from build123d import *

# Parameters (mm, degrees)
BOSS_EXTRUDE1_DEPTH = 45
BOSS_EXTRUDE2_DEPTH = 45


with BuildPart() as part:
    # Sketch1 → Boss-Extrude1 (new body)
    with BuildSketch(Plane(origin=(0, 0, 0), x_dir=(1, 0, 0), z_dir=(0, 1, 0))):
        Polygon((10.257365227, -10.154791575), (13.922990088, 3.805743075), (3.66562486, 13.96053465), (-10.257365227, 10.154791575), (-13.922990088, -3.805743075), (-3.66562486, -13.96053465), align=None)
        Polygon((-2.785874894, -10.610006334), (7.795597573, -7.717641597), (10.581472467, 2.892364737), (2.785874894, 10.610006334), (-7.795597573, 7.717641597), (-10.581472467, -2.892364737), align=None, mode=Mode.SUBTRACT)
    extrude(amount=BOSS_EXTRUDE1_DEPTH)

    # Sketch2 → Boss-Extrude2 (add)
    with BuildSketch(Plane(origin=(0, 45, 0), x_dir=(1, 0, 0), z_dir=(0, 1, 0))):
        Polygon((-6.68367368, -6.751185536), (1.391190433, 10.228779981), (2.592952284, 10.557272411), (-5.972802955, -7.454947554), align=None)
        Polygon((2.504861339, -9.163823965), (3.684441387, 9.720425506), (2.928005116, 10.469297414), (1.68769549, -9.387190014), align=None)
    extrude(amount=-BOSS_EXTRUDE2_DEPTH)


solid = part.part
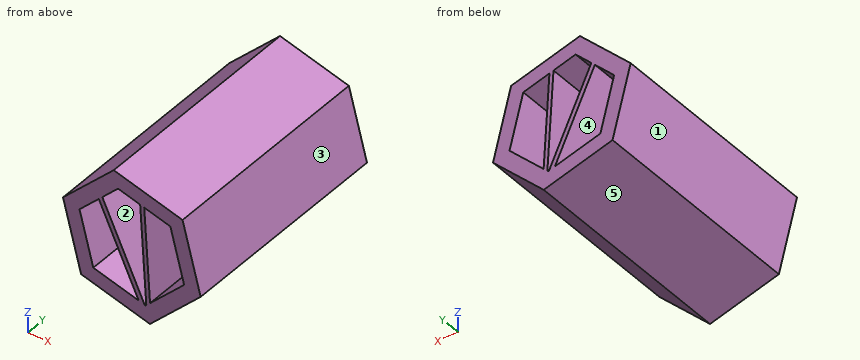
The model under review builds one solid part; all positions refer to its coordinate system, in mm. Face numbers are marked on the shaded views. A direction names the side the tool comes from. Round coordinates to 2 decimals unless told otherwise and drop trailing zeros. Loops run counter-clockwise (first coordinate to the right, second up) from the corner with the lowest first, then second, coordinate; pieces in that order, holes last. Notation, with made-up numbers: (73.25, 75.25) -> (86.25, 75.25) arc R21 cw to (86.25, 103.25) -> close; hole circle Ø2 at (15, 37.25). An arc over 180 degrees is marked (long way). Write item = value, one per line. Start each with the question number.
Item 1: Take a section at D-D on z = -6.5. Give the boundary of the cut face in (x, y).
Item 2: For the marked faces 4 and 5, list the 3-axis set-ups (+Z, -Z, +X, -X, +Y, -Y) from which the entire face can be reached by the end or side of a thin tool; tool diameter is ignored.
Item 3: Mouldability with a two-part tool opening along X and no side actions: class the marked faces 1, 2 and 3 as released by +X, released by -X, zero draft, split by the parting line, or undercut.
Item 4: Take a section at A-A on x = -1.5. Give the boundary of the cut face in (y, z), plus the area to 3 significant figures.
Item 5: Insertion check: pin 1 (12 mm diameter, centred on y = 8, z = 2.5, fed in from -X); pin 2 (6 mm diameter, centred on x = 1, y = 4.5, fed in from +Z); pin 3 (12 mm diameter, centred on x = 7.5, y = 40, fed in from -Z). Each pin has a flat end and moves straight along its axis. Give the tip position at first contact, or say it passes through.
Item 6: Take a section at C-C on y = 13.5. Give the boundary of the cut face in (x, z).
Item 7: Take a section at B-B on z = -1.75. Give the boundary of the cut face in (x, y).
Item 8: To check wall thickness, follow L1, parallel to X at y = 22.5, z = -3.75; L2, parallel to X at y = 39, z = -4; L3, parallel to Z at x = 7.5, y = 42. State the ranges of each line that lie inside material, in increasing order.
Result:
q1.outline = (-11.22, 0) -> (-8.12, 0) -> (-8.12, 45) -> (-11.22, 45) -> close; (-0.38, 0) -> (0.66, 0) -> (0.66, 45) -> (-0.38, 45) -> close; (2.68, 0) -> (3.48, 0) -> (3.48, 45) -> (2.68, 45) -> close; (6.94, 0) -> (11.2, 0) -> (11.2, 45) -> (6.94, 45) -> close
q2.face_4 = +Y, -Y
q2.face_5 = -Z, -X, +Y, -Y
q3.face_1 = released by -X
q3.face_2 = undercut
q3.face_3 = released by +X
q4.outline = (0, -12.55) -> (45, -12.55) -> (45, -9.44) -> (0, -9.44) -> close; (0, -4.15) -> (45, -4.15) -> (45, -1.95) -> (0, -1.95) -> close; (0, 10.26) -> (45, 10.26) -> (45, 13.37) -> (0, 13.37) -> close
q4.area = 379 mm²
q5.pin_1 = -13.92
q5.pin_2 = 13.51
q5.pin_3 = -13.96
q6.outline = (-13.92, 3.81) -> (-10.26, -10.15) -> (3.67, -13.96) -> (13.92, -3.81) -> (10.26, 10.15) -> (-3.67, 13.96) -> close; hole (-10.58, 2.89) -> (-7.8, -7.72) -> (1.39, -10.23) -> (-6.68, 6.75) -> close; hole (-5.97, 7.45) -> (2.59, -10.56) -> (2.79, -10.61) -> (2.93, -10.47) -> (1.69, 9.39) -> (-2.79, 10.61) -> close; hole (2.5, 9.16) -> (3.68, -9.72) -> (10.58, -2.89) -> (7.8, 7.72) -> close
q7.outline = (-12.46, 0) -> (-9.36, 0) -> (-9.36, 45) -> (-12.46, 45) -> close; (-2.64, 0) -> (-1.6, 0) -> (-1.6, 45) -> (-2.64, 45) -> close; (2.38, 0) -> (3.19, 0) -> (3.19, 45) -> (2.38, 45) -> close; (10.28, 0) -> (13.38, 0) -> (13.38, 45) -> (10.28, 45) -> close
q8.L1 = -11.94 to -8.84, -1.69 to -0.64, 2.51 to 3.31, 9.72 to 13.91
q8.L2 = -11.87 to -8.77, -1.57 to -0.53, 2.52 to 3.33, 9.46 to 13.73
q8.L3 = -10.16 to -5.94, 7.8 to 10.91
